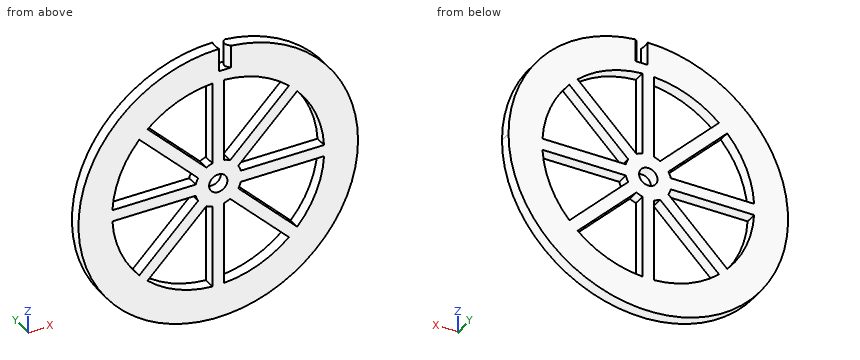
```python
from build123d import *

# Parameters (mm, degrees)
SKETCH1_R           = 76.2
SKETCH1_R_2         = 57.785
SKETCH1_R_3         = 12.7
SKETCH1_R_4         = 5
BOSS_EXTRUDE1_DEPTH = 3.175
CUT_EXTRUDE1_DEPTH  = 12.7


with BuildPart() as part:
    # Sketch1 → Boss-Extrude1 (new body, symmetric)
    with BuildSketch(Plane(origin=(0, 0, 0), x_dir=(1, 0, 0), z_dir=(0, 1, 0))):
        Circle(SKETCH1_R)
        Circle(SKETCH1_R_2, mode=Mode.SUBTRACT)
        with BuildLine():
            Line((-6.45003157, 10.940159631), (-38.553377116, 43.043505177))
            ThreePointArc((-38.553377116, 43.043505177), (-40.860165351, 40.860165351), (-43.043505177, 38.553377116))
            Line((-43.043505177, 38.553377116), (-10.940159631, 6.45003157))
            ThreePointArc((-10.940159631, 6.45003157), (-8.980256121, 8.980256121), (-6.45003157, 10.940159631))
        make_face()
        with BuildLine():
            Line((-12.296722124, 3.175), (-57.697708793, 3.175))
            ThreePointArc((-57.697708793, 3.175), (-57.785, 0), (-57.697708793, -3.175))
            Line((-57.697708793, -3.175), (-12.296722124, -3.175))
            ThreePointArc((-12.296722124, -3.175), (-12.7, 0), (-12.296722124, 3.175))
        make_face()
        with BuildLine():
            Line((-10.940159631, -6.45003157), (-43.043505177, -38.553377116))
            ThreePointArc((-43.043505177, -38.553377116), (-40.860165351, -40.860165351), (-38.553377116, -43.043505177))
            Line((-38.553377116, -43.043505177), (-6.45003157, -10.940159631))
            ThreePointArc((-6.45003157, -10.940159631), (-8.980256121, -8.980256121), (-10.940159631, -6.45003157))
        make_face()
        Circle(SKETCH1_R_3)
        Circle(SKETCH1_R_4, mode=Mode.SUBTRACT)
        with BuildLine():
            Line((-3.175, -12.296722124), (-3.175, -57.697708793))
            ThreePointArc((-3.175, -57.697708793), (0, -57.785), (3.175, -57.697708793))
            Line((3.175, -57.697708793), (3.175, -12.296722124))
            ThreePointArc((3.175, -12.296722124), (0, -12.7), (-3.175, -12.296722124))
        make_face()
        with BuildLine():
            ThreePointArc((38.553377116, -43.043505177), (40.860165351, -40.860165351), (43.043505177, -38.553377116))
            Line((43.043505177, -38.553377116), (10.940159631, -6.45003157))
            ThreePointArc((10.940159631, -6.45003157), (8.980256121, -8.980256121), (6.45003157, -10.940159631))
            Line((6.45003157, -10.940159631), (38.553377116, -43.043505177))
        make_face()
        with BuildLine():
            ThreePointArc((57.785, 0), (57.763173076, 1.588099867), (57.697708793, 3.175))
            Line((57.697708793, 3.175), (12.296722124, 3.175))
            ThreePointArc((12.296722124, 3.175), (12.598777143, 1.600254515), (12.7, 0))
            ThreePointArc((12.7, 0), (12.598777143, -1.600254515), (12.296722124, -3.175))
            Line((12.296722124, -3.175), (57.697708793, -3.175))
            ThreePointArc((57.697708793, -3.175), (57.763173076, -1.588099867), (57.785, 0))
        make_face()
        with BuildLine():
            ThreePointArc((43.043505177, 38.553377116), (40.860165351, 40.860165351), (38.553377116, 43.043505177))
            Line((38.553377116, 43.043505177), (6.45003157, 10.940159631))
            ThreePointArc((6.45003157, 10.940159631), (8.980256121, 8.980256121), (10.940159631, 6.45003157))
            Line((10.940159631, 6.45003157), (43.043505177, 38.553377116))
        make_face()
        with BuildLine():
            ThreePointArc((3.175, 57.697708793), (0, 57.785), (-3.175, 57.697708793))
            Line((-3.175, 57.697708793), (-3.175, 12.296722124))
            ThreePointArc((-3.175, 12.296722124), (0, 12.7), (3.175, 12.296722124))
            Line((3.175, 12.296722124), (3.175, 57.697708793))
        make_face()
    extrude(amount=BOSS_EXTRUDE1_DEPTH, both=True)

    # Sketch2 → Cut-Extrude1 (cut)
    with BuildSketch(Plane.XY.offset(76.2)):
        with BuildLine():
            Line((1.701477372, 6.35), (14.401477372, 6.35))
            add(Edge.make_bspline(
                [(14.401477372, 6.35), (-9.645577139, 0), (14.401477372, -6.35)],
                knots=[5.397827698, 5.397827698, 5.397827698, 7.168542916, 7.168542916, 7.168542916], degree=2, weights=[1, 0.633012702, 1]))
            Line((14.401477372, -6.35), (1.701477372, -6.35))
            ThreePointArc((1.701477372, -6.35), (0, 0), (1.701477372, 6.35))
        make_face()
    extrude(amount=-CUT_EXTRUDE1_DEPTH, mode=Mode.SUBTRACT)


solid = part.part
```
Verification items for the finished model (mm, model axes). Give positions to 0.01 mm unless a question says otherwise; leave off trailing zeros. Order: outer loops, then holes, each group sorted by start corner. A loop starts at its lowest first (then second) coordinate and runs counter-clockwise, first axis right, second up. Notation, with made-up numbers: M 85.25,12 L 121.25,12 A30 cw 121.25,40 Z; hole C -20.75,7 d6. An arc over 180 degrees is marked long. Return JSON: item names as keys, results as strings. Group by question number.
1) Scan lines: line 1 (X direction, y = 0.5, z = 0); line 2 (X direction, y = -1, z = -51.5) (3 decimals). Record each from-to range of solid material in increasing order.
2) Section check D-D on z = -66. Record the cut outline in (x, y) (3 decimals).
3) Section check A-A on x = -45.5. Record the cut outline in (y, z) (3 decimals), and give its area (3 significant figures).
4) Section check C-C on y = 1.5. Give the number of separate pieces and of enclosed holes in the cut face, and give its area (3 significant figures).
5) Go/stop test with flat-tipped pins: pin 1 Ø3 at (y, z) = (-0.5, 24) entering from -X; pin 2 Ø3 at (x, y) = (-52, -2) entering from -Z; pin 3 Ø1.9 at (y, z) = (-1, -34.5) entering from +X; pin 4 Ø8 at (x, z) = (0, 0) entering from -Y. Record where each tip stops, or that it passes through.
6) Section check B-B on x = -30. Record the cut outline in (y, z) (3 decimals).
Answer block:
{
 "1": {"line 1": "x = -76.2 to -5, 5 to 76.2", "line 2": "x = -56.162 to -26.208, -3.175 to 3.175, 26.208 to 56.162"},
 "2": {"outline": "M -38.085,-3.175 L 38.085,-3.175 L 38.085,3.175 L -38.085,3.175 Z"},
 "3": {"outline": "M -3.175,-61.124 L 3.175,-61.124 L 3.175,-35.621 L -3.175,-35.621 Z; M -3.175,-3.175 L 3.175,-3.175 L 3.175,3.175 L -3.175,3.175 Z; M -3.175,35.621 L 3.175,35.621 L 3.175,61.124 L -3.175,61.124 Z", "area": "364 mm^2"},
 "4": {"separate pieces": "1", "enclosed holes": "9", "area": "10,400 mm^2"},
 "5": {"pin 1": "stops at x = -72.8", "pin 2": "stops at z = -57.06", "pin 3": "stops at x = 68.42", "pin 4": "passes through"},
 "6": {"outline": "M -3.175,-70.046 L 3.175,-70.046 L 3.175,-49.387 L -3.175,-49.387 Z; M -3.175,-34.49 L 3.175,-34.49 L 3.175,-25.51 L -3.175,-25.51 Z; M -3.175,-3.175 L 3.175,-3.175 L 3.175,3.175 L -3.175,3.175 Z; M -3.175,25.51 L 3.175,25.51 L 3.175,34.49 L -3.175,34.49 Z; M -3.175,49.387 L 3.175,49.387 L 3.175,70.046 L -3.175,70.046 Z"}
}
